from build123d import *

# Parameters (mm, degrees)
SKETCH1_W           = 77.47
SKETCH1_H           = 63.5
BOSS_EXTRUDE1_DEPTH = 6.35
SKETCH2_R           = 2.1
CUT_EXTRUDE1_DEPTH  = 6.35
FILLET1_R           = 2.54
SKETCH3_R           = 1.5
CUT_EXTRUDE2_DEPTH  = 10.16


with BuildPart() as part:
    # Sketch1 → Boss-Extrude1 (new body)
    with BuildSketch(Plane(origin=(0, 0, 0), x_dir=(1, 0, 0), z_dir=(0, 1, 0))):
        with Locations((38.735, 31.75)):
            Rectangle(SKETCH1_W, SKETCH1_H)
        Polygon((23.33761346, 32.697540577), (23.33761346, 59.344124755), (54.982420655, 59.344124755), (54.982420655, 32.697540577), (69.85, 32.697540577), (69.85, 7.62), (7.62, 7.62), (7.62, 32.697540577), align=None, mode=Mode.SUBTRACT)
    extrude(amount=BOSS_EXTRUDE1_DEPTH)

    # Sketch2 → Cut-Extrude1 (cut)
    with BuildSketch(Plane(origin=(0, 6.35, 0), x_dir=(1, 0, 0), z_dir=(0, 1, 0))):
        with Locations(Location((3.175, 3.175, 0), (0, 0, 270))):
            Circle(SKETCH2_R)
        with Locations(Location((74.295, 3.175, 0), (0, 0, 270))):
            Circle(SKETCH2_R)
        with Locations(Location((74.295, 60.325, 0), (0, 0, 270))):
            Circle(SKETCH2_R)
    extrude(amount=-CUT_EXTRUDE1_DEPTH, mode=Mode.SUBTRACT)

    # Fillet1
    fillet1_edges = [part.edges().sort_by_distance(p)[0] for p in [
        (0, 3.175, 0),
        (0, 3.175, -63.5),
        (77.47, 3.175, -63.5),
        (77.47, 3.175, 0),
    ]]
    fillet(fillet1_edges, radius=FILLET1_R)

    # Sketch3 → Cut-Extrude2 (cut)
    with BuildSketch(Plane(origin=(0, 6.35, 0), x_dir=(1, 0, 0), z_dir=(0, 1, 0))):
        with Locations(Location((11.43, 55.88, 0), (0, 0, 270))):
            Circle(SKETCH3_R)
        with Locations(Location((62.23, 55.88, 0), (0, 0, 270))):
            Circle(SKETCH3_R)
    extrude(amount=-CUT_EXTRUDE2_DEPTH, mode=Mode.SUBTRACT)


solid = part.part
The model under review builds one solid part; all positions refer to its coordinate system, in mm. A direction names the side the tool comes from. Give positions to 0.01 mm unless a question says otherwise; leave off trailing zeros. Loops run counter-clockwise (first coordinate to the right, second up) from the corner with the lowest first, then second, coordinate; pieces in that order, holes last. Notation, with made-up numbers: (86.25, 67) -> (116.25, 67) arc R29 cw to (116.25, 104) -> close; hole circle Ø10 at (-18.5, 49). An arc over 180 degrees is marked (long way). Put each result on its own line as item: value. Start each with the question number.
1. We need section B-B on z = -41.5. State the section outline as (x, y) points, then the cut area to 3 significant figures.
2. For faces 1 (the face through (39, 3, -7.62)), 2 (the face through (21, 6.35, -39)), list the 3-axis set-ups (+Z, -Z, +X, -X, +Y, -Y) from which the entire face can be reached by the end or side of a thin tool; tool diameter is ignored.
3. We need section A-A on x = 11.43. State the section outline as (y, z) points.
4. We need section D-D on z = -55.88. State the section outline as (x, y) points.
5. We need section C-C on x = 66.5. State the section outline as (y, z) points, then the cut area to 3 significant figures.
6. Wall thickness on probe 1 along X at (y, z) = (4.5, -55.88); probe 2 along Z at (x, y) = (74.5, 5.25); probe 3 along Z at (x, y) = (54, 5): over which ranges is each line inside the solid? List them lowest first.
7. Mouldability with a two-part tool opening along X and no side actions: class faces 3 (the face through (7.62, 3, -20)), 4 (the face through (77.47, 3, -31)), 5 (the face through (0, 3, -31)), 6 (the face through (38, 3, 0)) as released by +X, released by -X, zero draft, split by the parting line, or undercut.
Determined:
1. outline: (0, 0) -> (23.34, 0) -> (23.34, 6.35) -> (0, 6.35) -> close; (54.98, 0) -> (77.47, 0) -> (77.47, 6.35) -> (54.98, 6.35) -> close
1. area: 291 mm^2
2. face 1: +Y, -Y
2. face 2: +Z, -Z, +X, -X, +Y
3. outline: (0, -63.5) -> (6.35, -63.5) -> (6.35, -57.38) -> (0, -57.38) -> close; (0, -54.38) -> (6.35, -54.38) -> (6.35, -32.7) -> (0, -32.7) -> close; (0, -7.62) -> (6.35, -7.62) -> (6.35, 0) -> (0, 0) -> close
4. outline: (0, 0) -> (9.93, 0) -> (9.93, 6.35) -> (0, 6.35) -> close; (12.93, 0) -> (23.34, 0) -> (23.34, 6.35) -> (12.93, 6.35) -> close; (54.98, 0) -> (60.73, 0) -> (60.73, 6.35) -> (54.98, 6.35) -> close; (63.73, 0) -> (77.47, 0) -> (77.47, 6.35) -> (63.73, 6.35) -> close
5. outline: (0, -63.5) -> (6.35, -63.5) -> (6.35, -32.7) -> (0, -32.7) -> close; (0, -7.62) -> (6.35, -7.62) -> (6.35, 0) -> (0, 0) -> close
5. area: 244 mm^2
6. probe 1: 0 to 9.93, 12.93 to 23.34, 54.98 to 60.73, 63.73 to 77.47
6. probe 2: -63.5 to -62.41, -58.24 to -5.26, -1.09 to 0
6. probe 3: -63.5 to -59.34, -7.62 to 0
7. face 3: undercut
7. face 4: released by +X
7. face 5: released by -X
7. face 6: zero draft
